from build123d import *

# Parameters (mm, degrees)
SKETCH_1_W          = 42
SKETCH_1_H          = 42
SKETCH_1_R          = 1.5
EXTRUDE_1_DEPTH     = 20
SKETCH_2_R          = 11
EXTRUDE_2_DEPTH     = 2
SKETCH_3_R          = 2.5
EXTRUDE_3_DEPTH     = 11
CUT_EXTRUDE_START   = -9
CUT_EXTRUDE_1_DEPTH = 9


with BuildPart() as part:
    # 草图1 → 凸台-拉伸1 (new body)
    with BuildSketch(Plane(origin=(0, 0, 0), x_dir=(1, 0, 0), z_dir=(0, 1, 0))):
        with Locations((21, 21)):
            Rectangle(SKETCH_1_W, SKETCH_1_H)
        with Locations(Location((5.5, 5.5, 0), (0, 0, 270))):
            Circle(SKETCH_1_R, mode=Mode.SUBTRACT)
        with Locations(Location((36.5, 5.5, 0), (0, 0, 270))):
            Circle(SKETCH_1_R, mode=Mode.SUBTRACT)
        with Locations(Location((36.5, 36.5, 0), (0, 0, 270))):
            Circle(SKETCH_1_R, mode=Mode.SUBTRACT)
        with Locations(Location((5.5, 36.5, 0), (0, 0, 270))):
            Circle(SKETCH_1_R, mode=Mode.SUBTRACT)
    extrude(amount=EXTRUDE_1_DEPTH)

    # 草图2 → 凸台-拉伸2 (add)
    with BuildSketch(Plane(origin=(0, 20, 0), x_dir=(1, 0, 0), z_dir=(0, 1, 0))):
        with Locations(Location((21, 21, 0), (0, 0, 270))):
            Circle(SKETCH_2_R)
    extrude(amount=EXTRUDE_2_DEPTH)

    # 草图3 → 凸台-拉伸3 (add)
    with BuildSketch(Plane(origin=(0, 22, 0), x_dir=(1, 0, 0), z_dir=(0, 1, 0))):
        with Locations(Location((21, 21, 0), (0, 0, 270))):
            Circle(SKETCH_3_R)
    extrude(amount=EXTRUDE_3_DEPTH)

    # 草图4 → 切除-拉伸1 (cut)
    with BuildSketch(Plane(origin=(0, 33, 0), x_dir=(1, 0, 0), z_dir=(0, 1, 0)).offset(CUT_EXTRUDE_START)):
        with BuildLine():
            Line((23, 22.5), (23, 21))
            Line((23, 21), (23, 19.5))
            ThreePointArc((23, 19.5), (23.371708245, 20.209430585), (23.5, 21))
            ThreePointArc((23.5, 21), (23.371708245, 21.790569415), (23, 22.5))
        make_face()
    extrude(amount=CUT_EXTRUDE_1_DEPTH, mode=Mode.SUBTRACT)


solid = part.part
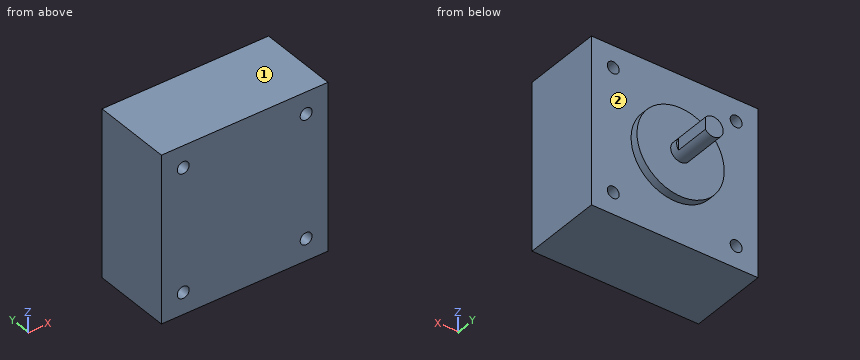
Check sheet for the modelled part. Datum: model origin and axes. Units: mm. Face numbers are marked on the shaded views. A direction names the side the tool comes from. Give positions to 0.01 mm unless a question says otherwise; leave off trailing zeros. Write each loop counter-clockwise with the first axis right and the second up, starting at its lowest first coordinate (ties: lowest second). Pieces come first, ordered by that corner, then holes. Notation, with made-up numbers: (40, -16) -> (77, -16) arc R9 ccw to (77, -2) -> close; hole circle Ø8 at (-21.5, 80.5). An arc over 180 degrees is marked (long way). One line per item, written item: value. Start each with the question number.
Item 1: Tool access check on the marked faces 1 and 2. Record the directions out of +Z, -Z, +X, -X, +Y, -Y that give a thin tool (end or side, any length) a straight path to the whole face; none if there is none.
Item 2: Section check A-A on z = -5.5. Record the cut outline in (x, y).
Item 3: Material ranges on probe 1 along X at (y, z) = (16.25, -5.5); probe 2 along X at (y, z) = (7, -5); probe 3 along Z at (x, y) = (5, 13), recorded low to high. Write a range as from..to.
Item 4: Section check C-C on y = 11. Record the cut outline in (x, z).
Item 5: Section check D-D on z = -21. Record the cut outline in (x, y).
Item 6: Section check B-B on x = 36.5. Record the cut outline in (y, z).
Item 7: Gauge pin test, flat ends, axial feed: pin 1 (5 mm diameter, centred on x = 5.5, z = -36.5, fed in from +Y); pin 2 (12 mm diameter, centred on x = 35, y = 28, fed in from -Z); pin 3 (2 mm diameter, centred on x = 16.5, z = -25.5, fed in from +Y); pin 4 (1.5 mm diameter, centred on y = 29, z = -21.5, fed in from +X). Record the tip position at first contact, or that the pin passes through.
Results list:
1. face 1: +Z, +X, -X, +Y, -Y
1. face 2: +Y
2. outline: (0, 0) -> (4, 0) -> (4, 20) -> (0, 20) -> close; (7, 0) -> (35, 0) -> (35, 20) -> (7, 20) -> close; (38, 0) -> (42, 0) -> (42, 20) -> (38, 20) -> close
3. probe 1: 0..4, 7..35, 38..42
3. probe 2: 0..4.09, 6.91..35.09, 37.91..42
3. probe 3: -42..-37.91, -35.09..-6.91, -4.09..0
4. outline: (0, -42) -> (42, -42) -> (42, 0) -> (0, 0) -> close; hole circle Ø3 at (5.5, -36.5); hole circle Ø3 at (5.5, -5.5); hole circle Ø3 at (36.5, -36.5); hole circle Ø3 at (36.5, -5.5)
5. outline: (0, 0) -> (42, 0) -> (42, 20) -> (32, 20) -> (32, 22) -> (23.5, 22) -> (23.5, 24) -> (23, 24) -> (23, 33) -> (18.5, 33) -> (18.5, 22) -> (10, 22) -> (10, 20) -> (0, 20) -> close
6. outline: (0, -42) -> (20, -42) -> (20, -38) -> (0, -38) -> close; (0, -35) -> (20, -35) -> (20, -7) -> (0, -7) -> close; (0, -4) -> (20, -4) -> (20, 0) -> (0, 0) -> close
7. pin 1: y = 20
7. pin 2: through
7. pin 3: y = 22
7. pin 4: x = 23
